```python
from build123d import *

# Parameters (mm, degrees)
F0_W     = 8.8552413508
F0_H     = 2.8463285416
F0_W_2   = 4.4276230037
F0_H_2   = 6.3251759857
F0_H_3   = 11.7015708238
F0_W_3   = 10.4365367442
F1_DEPTH = 38.1


with BuildPart() as f1:
    # F0 (on Right) → F1 (new body)
    with BuildSketch(Plane.YZ):
        Polygon((-14.5478984341, 21.1860537529), (6.9576902315, 21.1860537529), (6.9576902315, 24.664901197), (0, 24.664901197), (-8.8552413508, 24.664901197), (-14.5478984341, 24.664901197), align=None)
        with Locations((-4.4276206754, 26.0880654678)):
            Rectangle(F0_W, F0_H)
        Polygon((-19.6080375463, 0), (13.2828634232, 0), (13.2828634232, 21.1860537529), (6.9576902315, 21.1860537529), (-14.5478984341, 21.1860537529), (-19.6080375463, 21.1860537529), align=None)
        Polygon((8.8552413508, -16.132466495), (21.1893301457, -16.132466495), (21.1893301457, 0), (13.2828634232, 0), (-19.6080375463, 0), (-24.6681738645, 0), (-46.8062832952, 0), (-46.8062832952, -16.132466495), (-40.1648506522, -16.132466495), (-29.728313908, -16.132466495), (0, -16.132466495), align=None)
        Polygon((-46.8062832952, 0), (-24.6681738645, 0), (-24.6681738645, 21.1860537529), (-30.9933461249, 21.1860537529), (-35.4209691286, 21.1860537529), (-46.8062832952, 21.1860537529), align=None)
        with Locations((-33.2071576267, 24.3486417457)):
            Rectangle(F0_W_2, F0_H_2)
        with Locations((4.4276206754, -21.9832519069)):
            Rectangle(F0_W, F0_H_3)
        with Locations((-34.9465822801, -21.9832519069)):
            Rectangle(F0_W_3, F0_H_3)
    extrude(amount=F1_DEPTH)


solid = f1.part
```
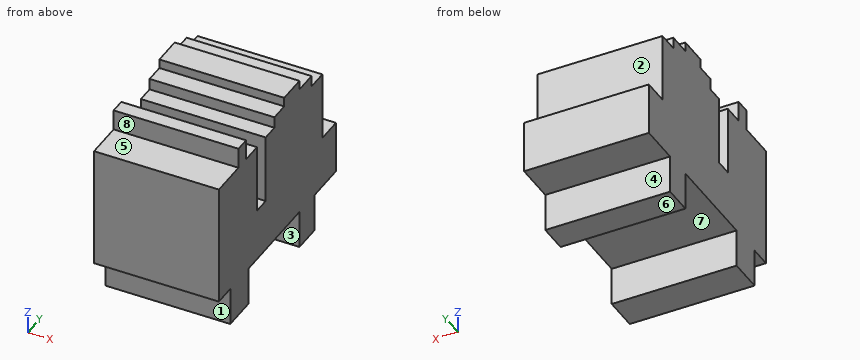
Geometry check sheet. Reference: the model listing, model coordinates, mm. Face numbers are marked on the shaded views. A direction names the side the tool comes from. Give positions to 0.01 mm unless a question says otherwise; leave off trailing zeros. Loops run counter-clockwise (first coordinate to the right, second up) from the corner with the lowest first, then second, coordinate; pieces in that order, holes last. Notation, with made-up numbers: M -39.5,-14.5 L -28.5,-14.5 A31 cw -28.5,21.5 Z; hole C -18.5,-9.5 d5. An arc over 180 degrees is marked long. Write item = value, one per line.
(1) Gauge pin test, flat ends, axial feed: pin 1 Ø3 at (x, y) = (27, -12) entering from +Z; pin 2 Ø5.5 at (x, y) = (19.5, -42.5) entering from +Z; pin 3 Ø1.7 at (x, z) = (28, 23.5) entering from -Y. Record the tip position at first contact, or that the pin passes through.
Answer below:
pin_1 = 24.66
pin_2 = 21.19
pin_3 = -35.42
(2) Tool access check on the marked faces 1, 2, 3, 4 and 5. Record the directions out of +Z, -Z, +X, -X, +Y, -Y that give a thin tool (end or side, any length) a straight path to the whole face; none if there is none.
Answer below:
face_1 = -Z, +X, -X, -Y
face_2 = +Z, +X, -X, +Y
face_3 = -Z, +X, -X
face_4 = -Z, +X, -X, +Y
face_5 = +Z, +X, -X, -Y
(3) Sectioned sample at A-A, the plane z = 22. Record the cut outline in (x, y), plus the area to 3 significant figures.
Answer below:
outline = M 0,-35.42 L 38.1,-35.42 L 38.1,-30.99 L 0,-30.99 Z; M 0,-14.55 L 38.1,-14.55 L 38.1,6.96 L 0,6.96 Z
area = 988 mm2
(4) Sectioned sample at C-C, the plane z = 2. Record the cut outline in (x, y).
Answer below:
outline = M 0,-46.81 L 38.1,-46.81 L 38.1,-24.67 L 0,-24.67 Z; M 0,-19.61 L 38.1,-19.61 L 38.1,13.28 L 0,13.28 Z
(5) Sectioned sample at D-D, the plane y = -16. Record the cut outline in (x, z), plus the area to 3 significant figures.
Answer below:
outline = M 0,-16.13 L 38.1,-16.13 L 38.1,21.19 L 0,21.19 Z
area = 1,420 mm2
(6) Material ranges on line 1 (Y direction, x = 11, z = 12); line 2 (Z direction, x = 17.5, y = 6.5); line 3 (Z direction, x = 7.5, y = -6), recorded low to high. Write a range as [from, to].
Answer below:
line_1 = [-46.81, -24.67], [-19.61, 13.28]
line_2 = [-27.83, 24.66]
line_3 = [-16.13, 27.51]
(7) Release check for a two-part mould opening along Y. For the marked faces 6, 7 and 8 record: released by +Y, released by -Y, zero draft, split by the parting line, or undercut.
Answer below:
face_6 = zero draft
face_7 = undercut
face_8 = released by -Y
